```python
from build123d import *

# Parameters (mm, degrees)
SZKIC4_R                   = 5.19169257
WYTNIJ_WYCI_GNI_CIE3_DEPTH = 12


with BuildPart() as part:
    # Szkic3 → Obr_t1 (revolve)
    with BuildSketch(Plane(origin=(0, 0, 0), x_dir=(0, 0, -1), z_dir=(1, 0, 0)), mode=Mode.PRIVATE) as obr_t1_sk:
        Polygon((0, 0), (0, 6.5), (1, 6.5), (1, 4.025), (24, 3.95), (24, 0), align=None)
    revolve(obr_t1_sk.sketch.rotate(Axis((0, 0, 0), (0, 0, -1)), 90), axis=Axis((0, 0, 0), (0, 0, -1)))

    # Szkic4 → Wytnij-wyci_gni_cie3 (cut)
    with BuildSketch(Plane(origin=(0, 0, -24), x_dir=(-1, 0, 0), z_dir=(0, 0, -1))):
        Circle(SZKIC4_R)
        Polygon((0, 3.810511777), (-3.3, 1.905255888), (-3.3, -1.905255888), (0, -3.810511777), (3.3, -1.905255888), (3.3, 1.905255888), align=None, mode=Mode.SUBTRACT)
    extrude(amount=-WYTNIJ_WYCI_GNI_CIE3_DEPTH, mode=Mode.SUBTRACT)


solid = part.part
```
For this review, take the finished solid that the model builds, in its own axes (mm). A direction names the side the tool comes from. Round coordinates to 2 decimals unless told otherwise and drop trailing zeros. Write each loop counter-clockwise with the first axis right and the second up, starting at its lowest first coordinate (ties: lowest second). Pieces come first, ordered by that corner, then holes. Notation, with made-up numbers: M 31.5,-39 L 70.5,-39 A15 ccw 70.5,-15 Z; hole C 15,83.5 d5. An arc over 180 degrees is marked long. One line per item, written item: value. Start each with the question number.
(1) Machinability: for faces 1 (the flat face through (-1.63, -2.87, -18.08)), 2 (the flat face through (1.673, -2.845, -18.084)), 3 (the flat face through (-3.3, 0, -18)), 4 (the flat face through (1.63, 2.87, -18.08)), 5 (the flat face through (3, -3, -1)), which of the approach directions +Z, -Z, +X, -X, +Y, -Y give a long, thin tool a straight path to every point of the face, cutting with its end or side? Answer none if there is none.
(2) Insertion check: pin 1 (3 mm diameter, centred on y = 0.5, z = -18.5, fed in from +X); pin 2 (3 mm diameter, centred on y = 0, z = -17.5, fed in from -X); pin 3 (3 mm diameter, centred on y = -2.5, z = -3.5, fed in from +X). Each pin has a flat end and moves straight along its axis. Give the tip position at first contact, or say it passes through.
(3) We need section C-C (z = -6.25). Give the boundary of the cut face in (x, y).
(4) Wall thickness on line 1 (Z direction, x = 4.75, y = -4); line 2 (Z direction, x = -3, y = -2.25); line 3 (X direction, y = -1.75, z = -19.25): over which ranges is each line inside the solid? List them lowest first.
(5) We need section A-A (z = -17). Give the boundary of the cut face in (x, y), and give its area (3 significant figures).
(6) We need section B-B (y = 5). Give the boundary of the cut face in (x, z).
Result:
1. face 1: -Z, -X, -Y
1. face 2: -Z, +X, -Y
1. face 3: -Z, -X, +Y, -Y
1. face 4: -Z, +X, +Y
1. face 5: -Z
2. pin 1: x = 3.3
2. pin 2: x = -3.3
2. pin 3: x = 3.89
3. outline: C 0,0 d8.02
4. line 1: -1 to 0
4. line 2: -12 to 0
4. line 3: -3.3 to 3.3
5. outline: M -3.3,-1.91 L 0,-3.81 L 3.3,-1.91 L 3.3,1.91 L 0,3.81 L -3.3,1.91 Z
5. area: 37.7 mm²
6. outline: M -4.15,-1 L 4.15,-1 L 4.15,0 L -4.15,0 Z
